```python
from build123d import *

# Parameters (mm, degrees)
F0_W     = 45.6249145791
F0_H     = 2.5061145425
F0_H_2   = 2.9115714133
F0_W_2   = 2.8638616204
F0_H_3   = 25.5405409262
F0_W_3   = 12.6152541488
F0_W_4   = 1.9348878413
F1_DEPTH = 25
F2_DEPTH = 25
F3_DEPTH = 25


with BuildPart() as f1:
    # F0 (on Top) → F1 (new body)
    with BuildSketch(Plane.XY):
        Polygon((-57.3309957981, 49.4364239275), (-59.3043640256, 49.4364239275), (-59.3043640256, 21.3805288076), (-59.3043640256, 8.8931322098), (-57.3309957981, 8.8931322098), (-57.3309957981, 46.9303093851), align=None)
        with Locations((-34.5185385086, 48.1833666563)):
            Rectangle(F0_W, F0_H)
        Polygon((39.7619791329, 49.4364239275), (-11.706081219, 49.4364239275), (-11.706081219, 46.9303093851), (-8.7652672082, 46.9303093851), (37.0916128159, 46.9303093851), (39.7619791329, 46.9303093851), align=None)
        Polygon((-57.3309957981, 8.8931322098), (-59.3043640256, 8.8931322098), (-59.3043640256, -42.6643118262), (-57.3309957981, -42.6643118262), (-57.3309957981, -39.752740413), (-57.3309957981, 6.6846082918), align=None)
        Polygon((70.7202106714, 49.4364239275), (39.7619791329, 49.4364239275), (39.7619791329, 46.9303093851), (67.856349051, 46.9303093851), (70.7202106714, 46.9303093851), align=None)
        with Locations((-34.5185385086, -41.2085261196)):
            Rectangle(F0_W, F0_H_2)
        Polygon((-8.7652672082, -61.8197210133), (-8.7652672082, -7.6428134926), (-11.706081219, -7.6428134926), (-11.706081219, -39.752740413), (-11.706081219, -42.6643118262), (-11.706081219, -61.8197210133), align=None)
        Polygon((70.7202106714, 46.9303093851), (67.856349051, 46.9303093851), (67.856349051, 22.3572142422), (67.856349051, 19.8326166719), (70.7202106714, 19.8326166719), align=None)
        Polygon((39.7619791329, -61.8197210133), (-8.7652672082, -61.8197210133), (-11.706081219, -61.8197210133), (-11.706081219, -64.0913546085), (55.2384853363, -64.0913546085), (55.2384853363, -61.8197210133), (53.3062070608, -61.8197210133), align=None)
        with Locations((69.2882798612, 7.0623462088)):
            Rectangle(F0_W_2, F0_H_3)
        with Locations((61.5487219766, 7.0623462088)):
            Rectangle(F0_W_3, F0_H_3)
        Polygon((53.3062070608, -23.8958857954), (53.3062070608, -61.8197210133), (55.2384853363, -61.8197210133), (55.2410949022, -61.8197210133), (55.2410949022, -5.7079242542), (53.3062070608, -5.7079242542), (53.3062070608, -20.9843106568), align=None)
        with Locations((54.2736509815, 7.0623462088)):
            Rectangle(F0_W_4, F0_H_3)
    extrude(amount=F1_DEPTH)

    # F0 (on Top) → F2 (join)
    with BuildSketch(Plane.XY):
        Polygon((-57.3309957981, 49.4364239275), (-59.3043640256, 49.4364239275), (-59.3043640256, 21.3805288076), (-59.3043640256, 8.8931322098), (-57.3309957981, 8.8931322098), (-57.3309957981, 46.9303093851), align=None)
        with Locations((-34.5185385086, 48.1833666563)):
            Rectangle(F0_W, F0_H)
        Polygon((39.7619791329, 49.4364239275), (-11.706081219, 49.4364239275), (-11.706081219, 46.9303093851), (-8.7652672082, 46.9303093851), (37.0916128159, 46.9303093851), (39.7619791329, 46.9303093851), align=None)
        Polygon((-57.3309957981, 8.8931322098), (-59.3043640256, 8.8931322098), (-59.3043640256, -42.6643118262), (-57.3309957981, -42.6643118262), (-57.3309957981, -39.752740413), (-57.3309957981, 6.6846082918), align=None)
        Polygon((70.7202106714, 49.4364239275), (39.7619791329, 49.4364239275), (39.7619791329, 46.9303093851), (67.856349051, 46.9303093851), (70.7202106714, 46.9303093851), align=None)
        with Locations((-34.5185385086, -41.2085261196)):
            Rectangle(F0_W, F0_H_2)
        Polygon((-8.7652672082, -61.8197210133), (-8.7652672082, -7.6428134926), (-11.706081219, -7.6428134926), (-11.706081219, -39.752740413), (-11.706081219, -42.6643118262), (-11.706081219, -61.8197210133), align=None)
        Polygon((70.7202106714, 46.9303093851), (67.856349051, 46.9303093851), (67.856349051, 22.3572142422), (67.856349051, 19.8326166719), (70.7202106714, 19.8326166719), align=None)
        Polygon((39.7619791329, -61.8197210133), (-8.7652672082, -61.8197210133), (-11.706081219, -61.8197210133), (-11.706081219, -64.0913546085), (55.2384853363, -64.0913546085), (55.2384853363, -61.8197210133), (53.3062070608, -61.8197210133), align=None)
        with Locations((69.2882798612, 7.0623462088)):
            Rectangle(F0_W_2, F0_H_3)
        with Locations((61.5487219766, 7.0623462088)):
            Rectangle(F0_W_3, F0_H_3)
        Polygon((53.3062070608, -23.8958857954), (53.3062070608, -61.8197210133), (55.2384853363, -61.8197210133), (55.2410949022, -61.8197210133), (55.2410949022, -5.7079242542), (53.3062070608, -5.7079242542), (53.3062070608, -20.9843106568), align=None)
        with Locations((54.2736509815, 7.0623462088)):
            Rectangle(F0_W_4, F0_H_3)
    extrude(amount=F2_DEPTH)

    # F0 (on Top) → F3 (join)
    with BuildSketch(Plane.XY):
        Polygon((-57.3309957981, 49.4364239275), (-59.3043640256, 49.4364239275), (-59.3043640256, 21.3805288076), (-59.3043640256, 8.8931322098), (-57.3309957981, 8.8931322098), (-57.3309957981, 46.9303093851), align=None)
        with Locations((-34.5185385086, 48.1833666563)):
            Rectangle(F0_W, F0_H)
        Polygon((39.7619791329, 49.4364239275), (-11.706081219, 49.4364239275), (-11.706081219, 46.9303093851), (-8.7652672082, 46.9303093851), (37.0916128159, 46.9303093851), (39.7619791329, 46.9303093851), align=None)
        Polygon((-57.3309957981, 8.8931322098), (-59.3043640256, 8.8931322098), (-59.3043640256, -42.6643118262), (-57.3309957981, -42.6643118262), (-57.3309957981, -39.752740413), (-57.3309957981, 6.6846082918), align=None)
        Polygon((70.7202106714, 49.4364239275), (39.7619791329, 49.4364239275), (39.7619791329, 46.9303093851), (67.856349051, 46.9303093851), (70.7202106714, 46.9303093851), align=None)
        with Locations((-34.5185385086, -41.2085261196)):
            Rectangle(F0_W, F0_H_2)
        Polygon((-8.7652672082, -61.8197210133), (-8.7652672082, -7.6428134926), (-11.706081219, -7.6428134926), (-11.706081219, -39.752740413), (-11.706081219, -42.6643118262), (-11.706081219, -61.8197210133), align=None)
        Polygon((70.7202106714, 46.9303093851), (67.856349051, 46.9303093851), (67.856349051, 22.3572142422), (67.856349051, 19.8326166719), (70.7202106714, 19.8326166719), align=None)
        Polygon((39.7619791329, -61.8197210133), (-8.7652672082, -61.8197210133), (-11.706081219, -61.8197210133), (-11.706081219, -64.0913546085), (55.2384853363, -64.0913546085), (55.2384853363, -61.8197210133), (53.3062070608, -61.8197210133), align=None)
        with Locations((69.2882798612, 7.0623462088)):
            Rectangle(F0_W_2, F0_H_3)
        with Locations((61.5487219766, 7.0623462088)):
            Rectangle(F0_W_3, F0_H_3)
        Polygon((53.3062070608, -23.8958857954), (53.3062070608, -61.8197210133), (55.2384853363, -61.8197210133), (55.2410949022, -61.8197210133), (55.2410949022, -5.7079242542), (53.3062070608, -5.7079242542), (53.3062070608, -20.9843106568), align=None)
        with Locations((54.2736509815, 7.0623462088)):
            Rectangle(F0_W_4, F0_H_3)
    extrude(amount=F3_DEPTH)


solid = f1.part
```
Here's how the part is built. I have some questions about the finished solid (model axes, mm). A direction names the side the tool comes from. Coordinates: 2 decimals unless noted, no trailing zeros. Write each loop counter-clockwise with the first axis right and the second up, starting at its lowest first coordinate (ties: lowest second). Pieces come first, ordered by that corner, then holes. Notation, with made-up numbers: (70.5, 59) -> (94.5, 59) arc R15 cw to (94.5, 78) -> close; hole circle Ø3 at (32, 69.25). An arc over 180 degrees is marked (long way). Use a Markdown table: item, result. Add a question column.
(1) Please list where these lines run through material, in increasing order: line 1 (X direction, y = -14.5, z = 23.5); line 2 (X direction, y = 28.5, z = 3); line 3 (Y direction, x = -53.5, z = 7.5).
(2) If we section it at B-B, the plane y = -12: Write out the boundary of the cut face in (x, z).
(3) If we section it at C-C, the plane y = -57: Write out the boundary of the cut face in (x, z), and give its area (3 significant figures).
(4) For faces 4 (the flat face through (63, -5.708, 12)), 5 (the flat face through (-59.304, 4, 12)), 6 (the flat face through (-36, -42.664, 12)), 7 (the flat face through (61, 19.833, 12)), which set-ups out of +Z, -Z, +X, -X, +Y, -Y let a thin tool reach every point of the face, with its end or its side?
(5) I'm going to push flat-ended pins straight in: P1, Ø12.5, axis at x = -27.5, z = 8, coming from the -Y side; P2, Ø7.5, axis at y = -22, z = 6.5, coming from the +X side; P3, Ø6.5, axis at y = -53, z = 6.5, coming from the -X side. Where does each tip first touch, or does it pass through?
(6) We'd pull the mould along X, two halves only. Please class faces 1 (the flat face through (-10, -7.643, 12)), 2 (the flat face through (54, 6, 25)), 3 (the flat face through (55.241, -34, 12)): +X half, -X half, draft (parallel to the pull), parting line (faces both ways), or undercut.
(7) If we section it at A-A, the plane x = 36: Write out the boundary of the cut face in (y, z).
Outcome:
| question | item | result |
|---|---|---|
| 1 | line 1 | x = -59.3 to -57.33, -11.71 to -8.77, 53.31 to 55.24 |
| 1 | line 2 | x = -59.3 to -57.33, 67.86 to 70.72 |
| 1 | line 3 | y = -42.66 to -39.75, 46.93 to 49.44 |
| 2 | outline | (-59.3, 0) -> (-57.33, 0) -> (-57.33, 25) -> (-59.3, 25) -> close; (-11.71, 0) -> (-8.77, 0) -> (-8.77, 25) -> (-11.71, 25) -> close; (53.31, 0) -> (55.24, 0) -> (55.24, 25) -> (53.31, 25) -> close |
| 3 | outline | (-11.71, 0) -> (-8.77, 0) -> (-8.77, 25) -> (-11.71, 25) -> close; (53.31, 0) -> (55.24, 0) -> (55.24, 25) -> (53.31, 25) -> close |
| 3 | area | 122 mm^2 |
| 4 | face 4 | +Z, -Z, +X, -Y |
| 4 | face 5 | +Z, -Z, -X, +Y, -Y |
| 4 | face 6 | +Z, -Z, -X, -Y |
| 4 | face 7 | +Z, -Z |
| 5 | P1 | stops at y = -42.66 |
| 5 | P2 | stops at x = 55.24 |
| 5 | P3 | stops at x = -11.71 |
| 6 | face 1 | undercut |
| 6 | face 2 | draft |
| 6 | face 3 | +X half |
| 7 | outline | (-64.09, 0) -> (-61.82, 0) -> (-61.82, 25) -> (-64.09, 25) -> close; (46.93, 0) -> (49.44, 0) -> (49.44, 25) -> (46.93, 25) -> close |
